Autodesk Inventor part; units mm, degrees
ref_plane "Start Plane" through (0, 0, 0) normal (0, 0, 1) x (1, 0, 0)
ref_plane "End Plane" through (0, 0, 240) normal (0, 0, 1) x (1, 0, 0)
ref_plane "Work Plane11" through (-11.9502, 8.0498, 240) normal (0.7071, 0, 0.7071) x (0.7071, 0, -0.7071)
ref_plane "Start Plane" through (0, 0, 0) normal (0, 0, 1) x (1, 0, 0)
ref_plane "End Plane" through (0, 0, 240) normal (0, 0, 1) x (1, 0, 0)
sketch "Sketch" plane through (0, 0, 0) normal (0, 0, 1) x (1, 0, 0)
  line L0 (-5.9502, 0.0498) -> (-5.9502, 25.6498)
  line L1 (-11.9502, 28.0498) -> (-8.3502, 28.0498)
  line L2 (-11.9502, -11.9502) -> (-11.9502, 28.0498)
  line L3 (-11.9502, -11.9502) -> (28.0498, -11.9502)
  line L4 (28.0498, -8.3502) -> (28.0498, -11.9502)
  line L5 (0.0498, -5.9502) -> (25.6498, -5.9502)
  arc A0 (-5.9502, 0.0498) -> (0.0498, -5.9502) centre (0.0498, 0.0498) ccw
  arc A1 (-5.9502, 25.6498) -> (-8.3502, 28.0498) centre (-8.3502, 25.6498) ccw
  arc A2 (28.0498, -8.3502) -> (25.6498, -5.9502) centre (25.6498, -8.3502) ccw
  line L6 (0, 36.6463) -> (0, -20.0496) construction
  line L7 (-20.0496, 0) -> (36.6463, 0) construction
  point P0 (-5.9502, -5.9502)
  point P1 (-5.9502, 28.0498)
  point P2 (28.0498, -5.9502)
  dimension "d4" = 40
  dimension "d6" = 40
  dimension "d8" = 6
  dimension "d10" = 6
  dimension "d17" = 6
  dimension "d18" = 2.4
  dimension "d19" = 11.9502
  dimension "d20" = 11.9502
extrude "Body" add sketch "Sketch" along normal up to surface (240 mm away) from surface at 0
sketch "Sketch3" plane through (0, 0, 0) normal (0, 0, 1) x (1, 0, 0)
  line L0 (0, 0) -> (10, 0)
ref_plane "Work Plane10" through (0, 0, 0) normal (0, -1, 0) x (1, 0, 0)
sketch "Sketch4" plane through (0, 0, 0) normal (0, -1, 0) x (1, 0, 0)
  line L0 (-2, 0) -> (12, 0)
  line L1 (-2, 240) -> (12, 240)
  dimension "d24" = 240
ref_plane "Work Plane11" through (-11.9502, 8.0498, 240) normal (0.7071, 0, 0.7071) x (0.7071, 0, -0.7071)
split "Split1" plane through (-11.9502, 8.0498, 240) removes the side toward (0.7071, 0, 0.7071)
ref_plane "Work Plane12" through (-11.9502, 8.0498, 0) normal (0.7071, 0, -0.7071) x (-0.7071, 0, -0.7071)
split "Split2" plane through (-11.9502, 8.0498, 0) removes the side toward (0.7071, 0, -0.7071)
equation "\"d4\" = b"
equation "\"d6\" = b"
equation "\"d17\" = R"
equation "\"d18\" = R1"
equation "\"d19\" = ex"
equation "\"d20\" = d19"
equation "\"d11\" = G_L"
equation "\"b\" = 40"
equation "\"ParT\" = 6"
equation "\"R\" = 6"
equation "\"R1\" = 2.4"
equation "\"G_L\" = d24"
equation "\"G_OFFSET_START\" = 0"
equation "\"G_OFFSET_END\" = 0"
properties part number "BS 4848 - 40x40x6-240" material "Steel, Mild"
Input: part model. Units: mm. Frame: model coordinates. A direction names the side the tool comes from. Give positions to 0.01 mm unless a question says otherwise; leave off trailing zeros. Order: outer loops, then holes, each group sorted by start corner. A loop starts at its lowest first (then second) coordinate and runs counter-clockwise, first axis right, second up. Notation, with made-up numbers: (-10, 20.5) -> (14, 20.5) arc R19 ccw to (14, 24.5) -> close; hole circle Ø7 at (5, 88). An arc over 180 degrees is marked (long way). Write each question's results on one line, items separated by ' | '. Start each with the question number.
Item 1: Set-up query: faces 1 (the flat face through (0.55, -6.86, 227.5)), 2 (the flat face through (-5.95, 13, 118)). Return all of +Z, -Z, +X, -X, +Y, -Y with unobstructed straight access to the full face (end or side cutting, diameter ignored); none if empty.
Item 2: Line query: line 1 (X direction, y = 3, z = 47); line 2 (X direction, y = -8, z = 175.5). Output: solid intervals per line, ascending.
Item 3: Contact query for flat-ended pins moving along their axis: P1, Ø1, axis at x = 21, z = 182.5, coming from the +Y side; P2, Ø13, axis at y = 17.5, z = 69.5, coming from the +X side; P3, Ø12, axis at x = -1, z = 190, coming from the +Y side. Output: stop coordinate, or through.
Item 4: Cut plane C-C on x = 18. Return the cut outline in (y, z), then the cut area to 3 significant figures.
Item 5: Cut plane A-A on z = 88.5. Return the cut outline in (x, y), then the cut area to 3 significant figures.
Item 6: Cut plane B-B on y = 16. Return the cut outline in (x, z), then the cut area to 3 significant figures.
Established:
1) face 1: +Z, +X, +Y, -Y | face 2: +Z, -Z, +X, +Y
2) line 1: -11.95 to -5.95 | line 2: -11.95 to 28.02
3) P1: y = -5.95 | P2: x = -5.95 | P3: y = 27.63
4) outline: (-11.95, 29.95) -> (-5.95, 29.95) -> (-5.95, 210.05) -> (-11.95, 210.05) -> close | area: 1,080 mm^2
5) outline: (-11.95, -11.95) -> (28.05, -11.95) -> (28.05, -8.35) arc R2.4 ccw to (25.65, -5.95) -> (0.05, -5.95) arc R6 cw to (-5.95, 0.05) -> (-5.95, 25.65) arc R2.4 ccw to (-8.35, 28.05) -> (-11.95, 28.05) -> close | area: 449 mm^2
6) outline: (-11.95, 0) -> (-5.95, 6) -> (-5.95, 234) -> (-11.95, 240) -> close | area: 1,400 mm^2
